from build123d import *

# Parameters (mm, degrees)
SKETCH_1_W          = 76.7
SKETCH_1_H          = 52.2
SKETCH_1_W_2        = 72.7
SKETCH_1_H_2        = 48.2
EXTRUDE_1_DEPTH     = 25
SKETCH_2_W          = 76.7
SKETCH_2_H          = 52.2
EXTRUDE_2_DEPTH     = 2
SKETCH_3_W          = 34.6
SKETCH_3_H          = 19.3
CUT_EXTRUDE_1_DEPTH = 2
SKETCH_4_W          = 36
SKETCH_4_H          = 34.3
CUT_EXTRUDE_2_DEPTH = 1
CHAMFER_1_SIZE      = 2
CUT_EXTRUDE_3_DEPTH = 2


with BuildPart() as part:
    # Эскиз1 → Бобышка-Вытянуть1 (new body)
    with BuildSketch(Plane(origin=(0, 0, 0), x_dir=(1, 0, 0), z_dir=(0, 1, 0))):
        with Locations((-18.59008079, -31.725044883)):
            Rectangle(SKETCH_1_W, SKETCH_1_H)
        with Locations((-18.59008079, -31.725044883)):
            Rectangle(SKETCH_1_W_2, SKETCH_1_H_2, mode=Mode.SUBTRACT)
    extrude(amount=EXTRUDE_1_DEPTH)

    # Эскиз2 → Бобышка-Вытянуть2 (add)
    with BuildSketch(Plane(origin=(0, 25, 0), x_dir=(1, 0, 0), z_dir=(0, 1, 0))):
        with Locations((-18.59008079, -31.725044883)):
            Rectangle(SKETCH_2_W, SKETCH_2_H)
    extrude(amount=EXTRUDE_2_DEPTH)

    # Эскиз3 → Вырез-Вытянуть1 (cut)
    with BuildSketch(Plane(origin=(0, 27, 0), x_dir=(1, 0, 0), z_dir=(0, 1, 0))):
        with Locations((-18.59008079, -31.725044883)):
            Rectangle(SKETCH_3_W, SKETCH_3_H)
    extrude(amount=-CUT_EXTRUDE_1_DEPTH, mode=Mode.SUBTRACT)

    # Эскиз4 → Вырез-Вытянуть2 (cut)
    with BuildSketch(Plane.XZ.offset(-25)):
        with Locations((-18.59008079, 31.725044883)):
            Rectangle(SKETCH_4_W, SKETCH_4_H)
    extrude(amount=-CUT_EXTRUDE_2_DEPTH, mode=Mode.SUBTRACT)

    # Фаска1
    chamfer_1_edges = [part.edges().sort_by_distance(p)[0] for p in [
        (-54.94008079, 25, 31.725044883),
        (-18.59008079, 25, 55.825044883),
        (17.75991921, 25, 31.725044883),
        (-18.59008079, 25, 7.625044883),
    ]]
    chamfer(chamfer_1_edges, length=CHAMFER_1_SIZE)

    # Эскиз5 → Вырез-Вытянуть3 (cut)
    with BuildSketch(Plane.ZY.offset(56.94008079)):
        with BuildLine():
            Line((35.628323132, 11.545750126), (35.628323132, 0))
            Line((35.628323132, 0), (27.128323132, 0))
            Line((27.128323132, 0), (27.128323132, 11.545750126))
            ThreePointArc((27.128323132, 11.545750126), (31.378323132, 15.795750126), (35.628323132, 11.545750126))
        make_face()
    extrude(amount=-CUT_EXTRUDE_3_DEPTH, mode=Mode.SUBTRACT)


solid = part.part
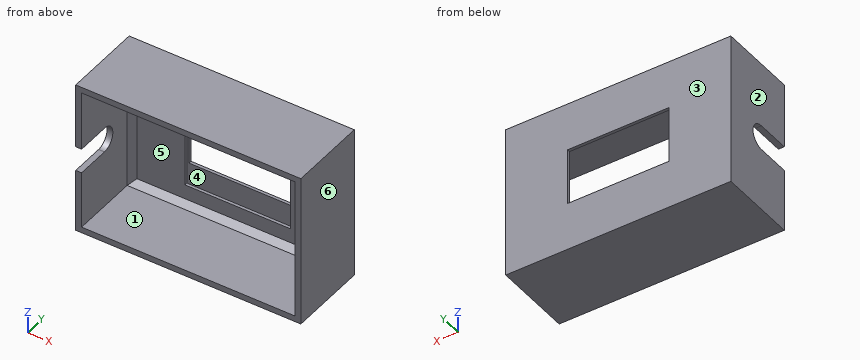
Work out the finished part from the listing and answer in its coordinate system (mm). Face numbers are marked on the shaded views. A direction names the side the tool comes from. Round coordinates to 2 decimals unless told otherwise and drop trailing zeros. Write each loop counter-clockwise with the first axis right and the second up, starting at its lowest first coordinate (ties: lowest second). Pieces come first, ordered by that corner, then holes. Notation, with made-up numbers: (29, -19.75) -> (82, -19.75) arc R16 cw to (82, -5.75) -> close; hole circle Ø11 at (61, 47.5). An arc over 180 degrees is marked (long way). Write each question's results on one line, items separated by ' | '.
Item 1: A flat-ended cylindrical pin translates along its axis: P1, Ø3, axis at x = 4.5, z = 23.5, coming from the -Y side. Find the tip coordinate at first contact, or state that the pin passes through.
Result set:
P1: y = 25
Item 2: Which of the six approach directions +Z, -Z, +X, -X, +Y, -Y give full straight-line access (tool end or side, diameter ignored) to the marked faces 5 and 6?
Result set:
face 5: -Y | face 6: +Z, -Z, +X, +Y, -Y
Item 3: The mould has two halves that part along X. Classify the marked faces 1, 2, 3 and 4: +X half, -X half, draft (parallel to the pull), parting line (faces both ways), or undercut.
Result set:
face 1: undercut | face 2: -X half | face 3: draft | face 4: undercut
Item 4: A cutting plane is placed at B-B, the plane y = 18. Determine the outline of the cut face in (x, z).
Result set:
outline: (-56.94, 5.63) -> (19.76, 5.63) -> (19.76, 57.83) -> (-56.94, 57.83) -> close; hole (-54.94, 7.63) -> (17.76, 7.63) -> (17.76, 55.83) -> (-54.94, 55.83) -> close
Item 5: Find the intervals of material crossed by line 1 along X through (y, z) = (21, 31); line 2 along Z through (x, y) = (-53, 11.5); line 3 along Y through (x, z) = (-33.5, 11), in increasing order. Write a range as [from, to].
Result set:
line 1: [-56.94, -54.94], [17.76, 19.76] | line 2: [5.63, 7.63], [55.83, 57.83] | line 3: [25, 27]
Item 6: A cutting plane is placed at C-C, the plane z = 24. Determine the outline of the cut face in (x, y).
Result set:
outline: (-56.94, 0) -> (-54.94, 0) -> (-54.94, 23) -> (-52.94, 25) -> (-36.59, 25) -> (-36.59, 26) -> (-35.89, 26) -> (-35.89, 27) -> (-56.94, 27) -> close; (-1.29, 26) -> (-0.59, 26) -> (-0.59, 25) -> (15.76, 25) -> (17.76, 23) -> (17.76, 0) -> (19.76, 0) -> (19.76, 27) -> (-1.29, 27) -> close
Item 7: A cutting plane is placed at D-D, the plane y = 3.75. Determine the outline of the cut face in (x, z), plus the area to 3 significant figures.
Result set:
outline: (-56.94, 5.63) -> (19.76, 5.63) -> (19.76, 57.83) -> (-56.94, 57.83) -> (-56.94, 35.63) -> (-54.94, 35.63) -> (-54.94, 55.83) -> (17.76, 55.83) -> (17.76, 7.63) -> (-54.94, 7.63) -> (-54.94, 27.13) -> (-56.94, 27.13) -> close | area: 483 mm^2
Item 8: A cutting plane is placed at A-A, the plane x = -18.5. Determine the outline of the cut face in (y, z), plus the area to 3 significant figures.
Result set:
outline: (0, 5.63) -> (27, 5.63) -> (27, 22.08) -> (26, 22.08) -> (26, 14.58) -> (25, 14.58) -> (25, 9.63) -> (23, 7.63) -> (0, 7.63) -> close; (0, 55.83) -> (23, 55.83) -> (25, 53.83) -> (25, 48.88) -> (26, 48.88) -> (26, 41.38) -> (27, 41.38) -> (27, 57.83) -> (0, 57.83) -> close | area: 155 mm^2
